Input: part model. Units: mm. Frame: model coordinates. Face numbers are marked on the shaded views. A direction names the side the tool comes from. Coordinates: 2 decimals unless noted, no trailing zeros. Write each loop counter-clockwise with the first axis right and the second up, starting at its lowest first coordinate (ties: lowest second). Pieces come first, ordered by that corner, then holes. Notation, with made-up numbers: (-19.5, -21) - (33.5, -21) arc R10 ccw to (33.5, -9) - close; hole circle Ø4 at (-20.5, -19). An arc over 180 degrees is marked (long way). One line per question, with ' | ' between items. Start each with the question number.
1) Reachability of the marked faces 1, 2 and 3 from +Z, -Z, +X, -X, +Y, -Y: full face, straight path, thin tool, end or side. Return the list, or none.
2) Line query: line 1 (Y direction, x = -1.5, z = -32); line 2 (Z direction, x = 2.25, y = -2); line 3 (Y direction, x = 0, z = -29.5). Output: solid intervals per line, ascending.
3) Section query A-A on z = 15.5. Return loops of the section in (x, y) (3 decimals), and give its area (3 significant figures).
4) First-contact query: P1, Ø1.5, axis at y = -2, z = 15.5, coming from the +X side; P2, Ø2, axis at y = 2, z = 16.5, coming from the +X side. Flat tips, straight axial feed; report the tip coordinate or a pass-through.
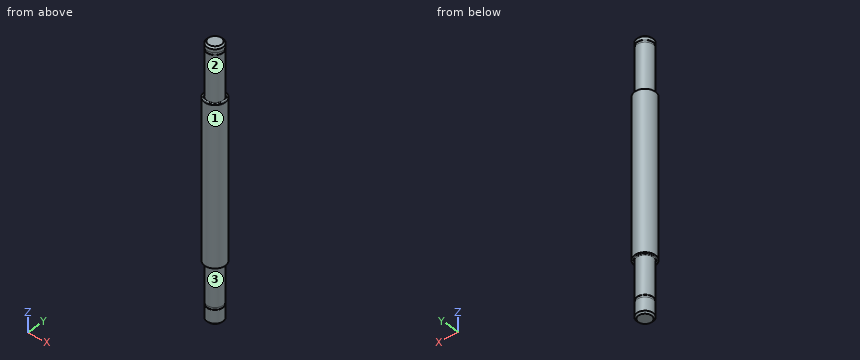
```python
from build123d import *

# Parameters (mm, degrees)
SKETCH1_R           = 2.5
BOSS_EXTRUDE1_DEPTH = 40.767
SKETCH2_W           = 0.7
SKETCH2_H           = 0.1
SKETCH5_R           = 3.175
BOSS_EXTRUDE3_DEPTH = 47.9552
SKETCH7_W           = 0.7
SKETCH7_H           = 0.1
CHAMFER1_SIZE       = 0.508
FILLET1_R           = 0.254


with BuildPart() as part:
    # Sketch1 → Boss-Extrude1 (new, symmetric)
    with BuildSketch(Plane.XY):
        with Locations(Location((0, 0, 0), (0, 0, 180))):
            Circle(SKETCH1_R)
    extrude(amount=BOSS_EXTRUDE1_DEPTH, both=True)

    # Sketch2 → Cut-Revolve1 (revolve, cut)
    with BuildSketch(Plane(origin=(0, 0, 0), x_dir=(0, 0, -1), z_dir=(1, 0, 0)), mode=Mode.PRIVATE) as cut_revolve1_sk:
        with Locations((-38.914555436, 2.45)):
            Rectangle(SKETCH2_W, SKETCH2_H)
    revolve(cut_revolve1_sk.sketch.rotate(Axis((0, 0, 40.767), (0, 0, -1)), 270), axis=Axis((0, 0, 40.767), (0, 0, -1)), mode=Mode.SUBTRACT)

    # Sketch5 → Boss-Extrude3 (add)
    with BuildSketch(Plane(origin=(0, 0, 24.364555436), x_dir=(-1, 0, 0), z_dir=(0, 0, -1))):
        with Locations(Location((0, 0, 0), (0, 0, 180))):
            Circle(SKETCH5_R)
    extrude(amount=BOSS_EXTRUDE3_DEPTH)

    # Sketch7 → Cut-Revolve2 (revolve, cut)
    with BuildSketch(Plane(origin=(0, -92.71594082, 0), x_dir=(0, 0, 1), z_dir=(1, 0, 0)), mode=Mode.PRIVATE) as cut_revolve2_sk:
        with Locations((-35.912002714, -95.16594082)):
            Rectangle(SKETCH7_W, SKETCH7_H)
    revolve(cut_revolve2_sk.sketch.rotate(Axis((0, 0, -23.590644564), (0, 0, -1)), 270), axis=Axis((0, 0, -23.590644564), (0, 0, -1)), mode=Mode.SUBTRACT)

    # Chamfer1
    chamfer1_edges = [part.edges().sort_by_distance(p)[0] for p in [
        (2.5, 0, -40.767),
        (2.5, 0, 40.767),
    ]]
    chamfer(chamfer1_edges, length=CHAMFER1_SIZE)

    # Fillet1
    fillet1_edges = [part.edges().sort_by_distance(p)[0] for p in [
        (2.5, 0, 24.364555436),
        (2.5, 0, -23.590644564),
    ]]
    fillet(fillet1_edges, radius=FILLET1_R)


solid = part.part
```
Answer key:
1) face 1: +Z, -Z | face 2: +Z | face 3: -Z
2) line 1: -2 to 2 | line 2: -23.59 to 24.36 | line 3: -2.5 to 2.5
3) outline: circle Ø6.35 at (0, 0) | area: 31.7 mm²
4) P1: x = 2.92 | P2: x = 3.01
